Autodesk Inventor part; units mm, degrees
ref_plane "YZ Plane" through (0, 0, 0) normal (1, 0, 0) x (0, 1, 0)
ref_plane "XZ Plane" through (0, 0, 0) normal (0, 1, 0) x (-1, 0, 0)
ref_plane "XY Plane" through (0, 0, 0) normal (0, 0, 1) x (1, 0, 0)
sketch "Sketch1" plane through (0, 0, 0) normal (0, 1, 0) x (-1, 0, 0)
  line L0 (0, 0) -> (-28.702, 0)
  line L1 (-28.702, 0) -> (-28.702, -66.04)
  line L2 (-28.702, -66.04) -> (0, -66.04)
  line L3 (0, -66.04) -> (0, 0)
  dimension "d0" = 28.702
  dimension "d1" = 66.04
extrude "Extrusion1" add sketch "Sketch1" along normal blind 3.048
sketch "Sketch2" plane through (0, 3.048, 0) normal (0, 1, 0) x (1, 0, 0)
  line L0 (0, 66.04) -> (0, 0)
  line L1 (28.702, 66.04) -> (0, 66.04)
  line L2 (0, 0) -> (2.54, 0)
  line L3 (2.54, 0) -> (2.54, 66.04)
  line L4 (2.54, 66.04) -> (0, 66.04)
  line L5 (0, 66.04) -> (0, 0)
  line L6 (28.702, 0) -> (28.702, 66.04)
  line L7 (28.702, 0) -> (2.54, 0)
  line L8 (2.54, 0) -> (2.54, 2.54)
  line L9 (2.54, 2.54) -> (28.702, 2.54)
  line L10 (28.702, 2.54) -> (28.702, 0)
  line L11 (2.54, 66.04) -> (28.702, 66.04)
  line L12 (28.702, 66.04) -> (28.702, 63.5)
  line L13 (28.702, 63.5) -> (2.54, 63.5)
  line L14 (2.54, 63.5) -> (2.54, 66.04)
  line L15 (28.702, 2.54) -> (26.162, 2.54)
  line L16 (26.162, 2.54) -> (26.162, 30.48)
  line L17 (26.162, 30.48) -> (28.702, 30.48)
  line L18 (28.702, 30.48) -> (28.702, 2.54)
  dimension "d4" = 2.54
  dimension "d5" = 2.54
  dimension "d6" = 2.54
  dimension "d7" = 2.54
  dimension "d8" = 27.94
extrude "Extrusion2" add sketch "Sketch2" along normal blind 40.64 contours L1 L3 L2 L0 | L1 L6 L13 L3 | L3 L9 L6 L7 | L16 L17 L6 L9
sketch "Sketch3" plane through (28.702, 0, -66.04) normal (0, 0, -1) x (-1, 0, 0)
  line L0 (28.702, 0) -> (23.622, 0)
  line L1 (23.622, 0) -> (23.622, 3.81)
  line L2 (23.622, 3.81) -> (28.702, 3.81)
  line L3 (28.702, 3.81) -> (28.702, 0)
  line L4 (23.622, 3.81) -> (10.922, 3.81)
  line L5 (10.922, 3.81) -> (10.922, 21.59)
  line L6 (10.922, 21.59) -> (23.622, 21.59)
  line L7 (23.622, 21.59) -> (23.622, 3.81)
  dimension "d11" = 5.08
  dimension "d12" = 3.81
  dimension "d13" = 12.7
  dimension "d14" = 17.78
extrude "Extrusion3" cut sketch "Sketch3" against normal blind 2.54 contours L4 L5 L6 L7
fillet "Fillet1" radius 6.35 4 edges at (17.78, 21.59, -64.77) (5.08, 21.59, -64.77) (5.08, 3.81, -64.77) (17.78, 3.81, -64.77)
properties part number "GoProCase"
CAD build for the part. Positions are in the model's coordinates, mm. A direction names the side the tool comes from. Coordinates: 2 decimals unless noted, no trailing zeros. Write each loop counter-clockwise with the first axis right and the second up, starting at its lowest first coordinate (ties: lowest second). Pieces come first, ordered by that corner, then holes. Notation, with made-up numbers: (-37.75, -1.5) -> (-25.75, -1.5) arc R19 ccw to (-25.75, 29.5) -> close; hole circle Ø3 at (-31.5, -2.75). An arc over 180 degrees is marked (long way). Use CSV: the item, a comma, the result in double quotes. Start each with the question number.
Item 1: Drop flat-ended pins along their axis: P1, Ø13, axis at x = 15, z = -21, coming from the +Y side; P2, Ø1, axis at y = 17, z = -47.5, coming from the +X side; P3, Ø2, axis at x = 13, y = 7.5, coming from the -Z side. Give the stop position or say it passes through.
Item 2: Band-saw the part on C-C, the plane z = -7.5. Write the cut outline in (x, y).
Item 3: Band-saw the part on A-A, the plane y = 14.5. Write the cut outline in (x, z).
Item 4: Tool access for faces 5 (the flat face through (27, 23, -30.48)), 6 (the flat face through (26.162, 23, -16)), 7 (the cylindrical face through (6.89, 5.72, -64.75)): list every direction of +Z, -Z, +X, -X, +Y, -Y with a clear straight run to the whole face (end or side of a thin tool).
Item 5: Band-saw the part on B-B, the plane x = 9.75. Write the cut outline in (y, z), plus the area to 3 significant figures.
Item 6: Band-saw the part on D-D, the plane x = 25. Write the cut outline in (y, z), plus the area to 3 significant figures.
Item 7: Two-plate mould, pull along Y, no slides. Class faces 1 (the flat face through (2.54, 23, -33)), 2 (the flat face through (5.08, 13, -65)), 3 (the flat face through (2, 43.688, -31)), 4 (the flat face through (17.78, 13, -65)): +Y half, -Y half, draft (parallel to the pull), parting line (faces both ways), or undercut.
Item 8: Wall check: probe 1 along Z at (x, y) = (5, 21); probe 2 along X at (y, z) = (9, -3); probe 3 along Z at (x, y) = (27, 21.5). Give the ranges that are in metal, low to high.
Response values:
1,P1,"stops at y = 3.05"
1,P2,"stops at x = 2.54"
1,P3,"stops at z = -2.54"
2,outline,"(0, 0) -> (28.7, 0) -> (28.7, 43.69) -> (26.16, 43.69) -> (26.16, 3.05) -> (2.54, 3.05) -> (2.54, 43.69) -> (0, 43.69) -> close"
3,outline,"(0, -66.04) -> (5.08, -66.04) -> (5.08, -63.5) -> (2.54, -63.5) -> (2.54, -2.54) -> (26.16, -2.54) -> (26.16, -30.48) -> (28.7, -30.48) -> (28.7, 0) -> (0, 0) -> close; (17.78, -66.04) -> (28.7, -66.04) -> (28.7, -63.5) -> (17.78, -63.5) -> close"
4,face 5,"+X, +Y"
4,face 6,"+Y"
4,face 7,"-Z"
5,outline,"(0, -66.04) -> (4.04, -66.04) -> (4.04, -63.5) -> (3.05, -63.5) -> (3.05, -2.54) -> (43.69, -2.54) -> (43.69, 0) -> (0, 0) -> close; (21.36, -66.04) -> (43.69, -66.04) -> (43.69, -63.5) -> (21.36, -63.5) -> close"
5,area,"364 mm2"
6,outline,"(0, -66.04) -> (43.69, -66.04) -> (43.69, -63.5) -> (3.05, -63.5) -> (3.05, -2.54) -> (43.69, -2.54) -> (43.69, 0) -> (0, 0) -> close"
6,area,"408 mm2"
7,face 1,"draft"
7,face 2,"undercut"
7,face 3,"+Y half"
7,face 4,"undercut"
8,probe 1,"z = -66.04 to -63.5, -2.54 to 0"
8,probe 2,"x = 0 to 2.54, 26.16 to 28.7"
8,probe 3,"z = -66.04 to -63.5, -30.48 to 0"
